```python
from build123d import *

# Parameters (mm, degrees)
F1_DEPTH = 600


with BuildPart() as f1:
    # F0 (on Top) → F1 (new body)
    with BuildSketch(Plane.XY):
        with BuildLine():
            ThreePointArc((-1.5, 0), (-1.06066, -1.06066), (0, -1.5))
            Line((0, -1.5), (47, -1.5))
            ThreePointArc((47, -1.5), (48.06066, -1.06066), (48.5, 0))
            Line((48.5, 0), (48.5, 18.5))
            Line((48.5, 18.5), (45.5, 18.5))
            Line((45.5, 18.5), (45.5, 4))
            ThreePointArc((45.5, 4), (44.767767, 2.232233), (43, 1.5))
            Line((43, 1.5), (4, 1.5))
            ThreePointArc((4, 1.5), (2.232233, 2.232233), (1.5, 4))
            Line((1.5, 4), (1.5, 18.5))
            Line((1.5, 18.5), (-1.5, 18.5))
            Line((-1.5, 18.5), (-1.5, 0))
        make_face()
    extrude(amount=F1_DEPTH)


solid = f1.part
```
Geometry check sheet. Reference: the model listing, model coordinates, mm. A direction names the side the tool comes from. Coordinates: 2 decimals unless noted, no trailing zeros. Write each loop counter-clockwise with the first axis right and the second up, starting at its lowest first coordinate (ties: lowest second). Pieces come first, ordered by that corner, then holes. Notation, with made-up numbers: M -24,62 L -10,62 A22 cw -10,79 Z; hole C 69,55 d10. An arc over 180 degrees is marked long. Use one line per item in the form item = value. Start each with the question number.
1) Section check B-B on z = 459.5. Enter the section's corners in (x, y), and give its area (3 significant figures).
2) Thickness scan on probe 1 along X at (y, z) = (4.25, 437); probe 2 along Y at (x, z) = (41.5, 156); probe 3 along X at (y, z) = (2.25, 281.5). Record the ranges inside material, lowest first. Write a range as from..to.
3) Set-up check for faces 1 (the flat face through (25, 1, 0)), 2 (the flat face through (45.5, 11, 296)): record each of +Z, -Z, +X, -X, +Y, -Y from which the full face is reachable in a straight line by a thin tool's end or side.
4) Go/stop test with a flat-tipped pin: pin 1 Ø6 at (x, z) = (7.5, 84) entering from +Y. Record where the tip stops, or that it passes through.
5) Section check A-A on y = 9.25. Enter the section's corners in (x, z).
6) Release check for a two-part mould opening along X. For faces 3 (the flat face through (48.5, 9, 296)), 4 (the flat face through (24, 1.5, 296)), 5 (the flat face through (-1.5, 9, 296)) record: pulls with the +X half, pulls with the -X half, needs draft (parallel to the pull), parting line crosses it, or undercut.
7) Section check C-C on x = 29.5. Enter the section's corners in (y, z).
Responses:
q1.outline = M -1.5,0 A1.5 ccw 0,-1.5 L 47,-1.5 A1.5 ccw 48.5,0 L 48.5,18.5 L 45.5,18.5 L 45.5,4 A2.5 cw 43,1.5 L 4,1.5 A2.5 cw 1.5,4 L 1.5,18.5 L -1.5,18.5 Z
q1.area = 254 mm2
q2.probe_1 = -1.5..1.5, 45.5..48.5
q2.probe_2 = -1.5..1.5
q2.probe_3 = -1.5..2.21, 44.79..48.5
q3.face_1 = -Z, +X, -X, +Y, -Y
q3.face_2 = +Z, -Z, +Y
q4.pin_1 = 1.5
q5.outline = M -1.5,0 L 1.5,0 L 1.5,600 L -1.5,600 Z; M 45.5,0 L 48.5,0 L 48.5,600 L 45.5,600 Z
q6.face_3 = pulls with the +X half
q6.face_4 = undercut
q6.face_5 = pulls with the -X half
q7.outline = M -1.5,0 L 1.5,0 L 1.5,600 L -1.5,600 Z
